Autodesk Inventor part; units mm, degrees
ref_plane "YZ Plane" through (0, 0, 0) normal (1, 0, 0) x (0, 1, 0)
ref_plane "XZ Plane" through (0, 0, 0) normal (0, 1, 0) x (-1, 0, 0)
ref_plane "XY Plane" through (0, 0, 0) normal (0, 0, 1) x (1, 0, 0)
sketch "Sketch1" plane through (0, 0, 0) normal (0, 0, 1) x (1, 0, 0)
  line L0 (0, 0) -> (25.4, 0)
  line L1 (25.4, 0) -> (25.4, 50.8)
  line L2 (25.4, 50.8) -> (0, 50.8)
  line L3 (0, 50.8) -> (0, 0)
  line L4 (1.5875, 1.5875) -> (23.8125, 1.5875)
  line L5 (23.8125, 1.5875) -> (23.8125, 49.2125)
  line L6 (23.8125, 49.2125) -> (1.5875, 49.2125)
  line L7 (1.5875, 49.2125) -> (1.5875, 1.5875)
  dimension "d0" = 25.4
  dimension "d1" = 50.8
  dimension "d2" = 1.5875
extrude "Extrusion1" add sketch "Sketch1" along normal mid plane 615.95
chamfer "Chamfer1" distance 25.4 angle 45 2 edges at (25.4, 25.4, 307.975) (25.4, 25.4, -307.975)
sketch "Sketch2" plane through (0, 0, 307.975) normal (-1, 0, 0) x (0, 0, 1)
  line L0 (-615.95, 0) -> (-615.95, 50.8)
  point P0 (-307.975, 0)
  point P1 (-307.975, 25.4)
  dimension "d8" = 25.4
  dimension "d9" = 307.975
hole "Hole1" at (0, 25.4, 0) direction (1, 0, 0) diameter 6.35 depth 25.4 tip angle 118 counterbore diameter 9.525 counterbore depth 6.35
properties part number "FRA_BackMainRail_002" material "Aluminum 6061"
Could you check a few things on this model? Use its own coordinates, in mm. A direction names the side the tool comes from. Give positions to 0.01 mm unless a question says otherwise; leave off trailing zeros. Loops run counter-clockwise (first coordinate to the right, second up) from the corner with the lowest first, then second, coordinate; pieces in that order, holes last. Notation, with made-up numbers: (22, 46.25) -> (42, 46.25) arc R9 ccw to (42, 53.25) -> close; hole circle Ø4 at (43, -11). An arc over 180 degrees is marked (long way). Return JSON: item names as keys, results as strings.
Item 1: If we section it at A-A on y = 36.5: List the corners of the cut face in (x, z) for me (1 decimal), plus the area to 4 significant figures.
Geometry results:
{"outline": "(0, -308) -> (1.6, -306.4) -> (1.6, 306.4) -> (0, 308) -> close; (23.8, -284.2) -> (25.4, -282.6) -> (25.4, 282.6) -> (23.8, 284.2) -> close", "area": "1,875 mm²"}
Item 2: If we section it at B-B on z = -138: List the corners of the cut face in (x, y) for me.
Geometry results:
{"outline": "(0, 0) -> (25.4, 0) -> (25.4, 50.8) -> (0, 50.8) -> close; hole (1.59, 1.59) -> (23.81, 1.59) -> (23.81, 49.21) -> (1.59, 49.21) -> close"}
Item 3: I need wall thicknesses on L1, parallel to Y at x = 6, z = -204; L2, parallel to X at y = 46.5, z = -250.5; L3, parallel to Y at x = 24.65, z = 0 (3 decimals). Which ranges of each line are inside material? Lowest first, please. Write a range as from..to.
Geometry results:
{"L1": "y = 0..1.59, 49.21..50.8", "L2": "x = 0..1.59, 23.81..25.4", "L3": "y = 0..22.225, 28.575..50.8"}
Item 4: We'd pull the mould along X, two halves only. Please class faces 4 (the flat face through (13, 1.588, -4)), 5 (the flat face through (25.4, 25, -4)), 6 (the flat face through (0, 20, -4)): +X half, -X half, draft (parallel to the pull), parting line (faces both ways), or undercut.
Geometry results:
{"face 4": "undercut", "face 5": "+X half", "face 6": "-X half"}
Item 5: If we section it at C-C on x = 17: List the corners of the cut face in (y, z) for me (1 decimal), plus the area to 3 significant figures.
Geometry results:
{"outline": "(0, -291) -> (1.6, -291) -> (1.6, 291) -> (0, 291) -> close; (49.2, -291) -> (50.8, -291) -> (50.8, 291) -> (49.2, 291) -> close", "area": "1,850 mm²"}
Item 6: I'm going to push a flat-ended pin straight in: pin 1 (6 mm diameter, centred on x = 16, y = 7.5, fed in from -Z). Where does the tip first touch, or does it pass through?
Geometry results:
{"pin 1": "passes through"}
Item 7: Which directions (+Z, -Z, +X, -X, +Y, -Y) give clear straight access to the entire face, cutting with the end or side of a thin tool? Please do faces 1 (the flat face through (13, 0, -4)), 2 (the flat face through (1.588, 31, -4)), 3 (the cylindrical face through (0.8, 20.68, -0.62)).
Geometry results:
{"face 1": "+Z, -Z, +X, -X, -Y", "face 2": "+Z, -Z", "face 3": "-X"}
